Check sheet for the modelled part. Datum: model origin and axes. Units: mm. A direction names the side the tool comes from. Give positions to 0.01 mm unless a question says otherwise; leave off trailing zeros. Write each loop counter-clockwise with the first axis right and the second up, starting at its lowest first coordinate (ties: lowest second). Pieces come first, ordered by that corner, then holes. Notation, with made-up numbers: M -18.75,-3.75 L 19.25,-3.75 A15 ccw 19.25,16.25 Z; hole C 65.25,34 d3. An arc over 180 degrees is marked long. Use CSV: the item, a comma, the result in double quotes. Start each with the question number.
1. Cross-section at A-A, the plane x = 5. Enter the section's corners in (y, z).
2. Access from +Z, -Z, +X, -X, +Y, -Y to the whole of each face (thin tool, end or side, straight path). Record for faces 1 (the face through (-151.18, 125.16, 2.81)), 2 (the face through (102.025, -153, 5)), 3 (the face through (-92.04, 60.52, 4.93)).
3. Scan lines: line 1 (X direction, y = -133.5, z = 7) (3 decimals); line 2 (X direction, y = -141, z = 7.25) (3 decimals); line 3 (X direction, y = 192, z = 1) (3 decimals). Record each from-to range of solid material in increasing order.
4. Depth check by flat-ended pin: P1, Ø2, axis at x = -58.5, z = 9, coming from the +Y side; P2, Ø3.5, axis at x = -117.025, z = 5, coming from the -Y side; P3, Ø8.5, axis at x = 148.52, y = -141, coming from the -Z side. Enter the tip coordinate at first touch or a pass-through.
from build123d import *

# Parameters (mm, degrees)
SALIENTE_EXTRUIR1_DEPTH                              = 10
PERFORADOR_PARA_ROSCAR_PARA_MACHO_DE_2_COUNT         = 2
PERFORADOR_PARA_ROSCAR_PARA_MACHO_DE_2_PITCH         = 50
PERFORADOR_PARA_ROSCAR_PARA_MACHO_DE_3_COUNT         = 2
PERFORADOR_PARA_ROSCAR_PARA_MACHO_DE_3_PITCH         = 114.274917137
PERFORADOR_PARA_ROSCAR_PARA_MACHO_DE_4_COUNT         = 2
PERFORADOR_PARA_ROSCAR_PARA_MACHO_DE_4_PITCH         = 25
PERFORADOR_PARA_ROSCAR_PARA_MACHO_DE_5_A_COUNT       = 2
PERFORADOR_PARA_ROSCAR_PARA_MACHO_DE_5_A_PITCH       = 50
PERFORADOR_PARA_ROSCAR_PARA_MACHO_DE_6_COUNT         = 2
PERFORADOR_PARA_ROSCAR_PARA_MACHO_DE_6_PITCH         = 24.875395913
REFRENTADO_PARA_TORNILLO_TAP_N_CON_CABEZ_D           = 5.3
REFRENTADO_PARA_TORNILLO_TAP_N_CON_CABEZ_CSINK_D     = 11.2
REFRENTADO_PARA_TORNILLO_TAP_N_CON_CABEZ_CSINK_ANGLE = 90
SIMETR_A3_COPY_1_D                                   = 5.3
SIMETR_A3_COPY_1_CSINK_D                             = 11.2
SIMETR_A3_COPY_1_CSINK_ANGLE                         = 90
CORTAR_EXTRUIR1_DEPTH                                = 286.71506895
CORTAR_EXTRUIR1_DEPTH_BACK                           = 286.71506895
CROQUIS8_R                                           = 4


with BuildPart() as part:
    # Croquis1 → Saliente-Extruir1 (new body)
    with BuildSketch(Plane.XY):
        with BuildLine():
            Line((-67.025, 50), (67.025, 50))
            ThreePointArc((67.025, 50), (91.773737342, 60.251262658), (102.025, 85))
            Line((102.025, 85), (102.025, 220))
            Line((102.025, 220), (182.025, 220))
            Line((182.025, 220), (182.025, 60))
            Line((182.025, 60), (182.025, -60))
            Line((182.025, -60), (182.025, -220))
            Line((182.025, -220), (102.025, -220))
            Line((102.025, -220), (102.025, -85))
            ThreePointArc((102.025, -85), (91.773737342, -60.251262658), (67.025, -50))
            Line((67.025, -50), (-67.025, -50))
            ThreePointArc((-67.025, -50), (-91.773737342, -60.251262658), (-102.025, -85))
            Line((-102.025, -85), (-102.025, -220))
            Line((-102.025, -220), (-182.025, -220))
            Line((-182.025, -220), (-182.025, -60))
            Line((-182.025, -60), (-182.025, 60))
            Line((-182.025, 60), (-182.025, 220))
            Line((-182.025, 220), (-102.025, 220))
            Line((-102.025, 220), (-102.025, 85))
            ThreePointArc((-102.025, 85), (-91.773737342, 60.251262658), (-67.025, 50))
        make_face()
    extrude(amount=SALIENTE_EXTRUIR1_DEPTH)

    # Croquis3 → Perforador para roscar para macho de ros (revolve, cut)
    with BuildSketch(Plane(origin=(-167.025, 220, 5), x_dir=(0, 0, 1), z_dir=(1, 0, 0))):
        Polygon((0, 0), (0, 76.2618073), (2.1, 75), (2.1, 0), align=None)
    perforador_para_roscar_para_macho_de_ros = revolve(axis=Axis((-167.025, 226.35, 5), (0, -1, 0)), mode=Mode.SUBTRACT)

    # Perforador para roscar para macho de 2: Perforador para roscar para macho de ros ×2
    with Locations(*[(i * PERFORADOR_PARA_ROSCAR_PARA_MACHO_DE_2_PITCH, 0, 0) for i in range(1, PERFORADOR_PARA_ROSCAR_PARA_MACHO_DE_2_COUNT)]):
        add(perforador_para_roscar_para_macho_de_ros, mode=Mode.SUBTRACT)

    # Perforador para roscar para macho de 3: Perforador para roscar para macho de ros ×2
    with Locations(*[Vector(-0.9105437359751597, 0, -0.4134127536450694) * (i * PERFORADOR_PARA_ROSCAR_PARA_MACHO_DE_3_PITCH) for i in range(1, PERFORADOR_PARA_ROSCAR_PARA_MACHO_DE_3_COUNT)]):
        add(perforador_para_roscar_para_macho_de_ros, mode=Mode.SUBTRACT)

    # Perforador para roscar para macho de 4: Perforador para roscar para macho de ros ×2
    with Locations(*[(i * PERFORADOR_PARA_ROSCAR_PARA_MACHO_DE_4_PITCH, 0, 0) for i in range(1, PERFORADOR_PARA_ROSCAR_PARA_MACHO_DE_4_COUNT)]):
        add(perforador_para_roscar_para_macho_de_ros, mode=Mode.SUBTRACT)

    # Croquis5 → Perforador para roscar para macho de 5 (revolve, cut)
    with BuildSketch(Plane(origin=(117.025, 220, 5), x_dir=(0, 0, 1), z_dir=(1, 0, 0))):
        Polygon((0, 0), (0, 76.2618073), (2.1, 75), (2.1, 0), align=None)
    perforador_para_roscar_para_macho_de_5 = revolve(axis=Axis((117.025, 226.35, 5), (0, -1, 0)), mode=Mode.SUBTRACT)

    # Perforador para roscar para macho de 5 a: Perforador para roscar para macho de 5 ×2
    with Locations(*[(i * PERFORADOR_PARA_ROSCAR_PARA_MACHO_DE_5_A_PITCH, 0, 0) for i in range(1, PERFORADOR_PARA_ROSCAR_PARA_MACHO_DE_5_A_COUNT)]):
        add(perforador_para_roscar_para_macho_de_5, mode=Mode.SUBTRACT)

    # Perforador para roscar para macho de 6: Perforador para roscar para macho de 5 ×2
    with Locations(*[Vector(0.9999846303252095, 0, 0.005544286550521713) * (i * PERFORADOR_PARA_ROSCAR_PARA_MACHO_DE_6_PITCH) for i in range(1, PERFORADOR_PARA_ROSCAR_PARA_MACHO_DE_6_COUNT)]):
        add(perforador_para_roscar_para_macho_de_5, mode=Mode.SUBTRACT)

    # Simetría1: Perforador para roscar para macho de ros, Perforador para roscar para macho de 5 across plane
    add(perforador_para_roscar_para_macho_de_ros.mirror(Plane.ZX), mode=Mode.SUBTRACT)
    add(perforador_para_roscar_para_macho_de_5.mirror(Plane.ZX), mode=Mode.SUBTRACT)

    # Simetría1 copy 1 sketch → Simetría1 copy 1 (revolve, cut)
    with BuildSketch(Plane(origin=(-117.025, -220, 5), x_dir=(0, 0, 1), z_dir=(1, 0, 0))):
        Polygon((0, 0), (0, -76.2618073), (2.1, -75), (2.1, 0), align=None)
    revolve(axis=Axis((-117.025, -226.35, 5), (0, -1, 0)), mode=Mode.SUBTRACT)

    # Simetría1 copy 2 sketch → Simetría1 copy 2 (revolve, cut)
    with BuildSketch(Plane(origin=(-271.077309978, -220, -42.242708166), x_dir=(0, 0, 1), z_dir=(1, 0, 0))):
        Polygon((0, 0), (0, -76.2618073), (2.1, -75), (2.1, 0), align=None)
    revolve(axis=Axis((-271.077309978, -226.35, -42.242708166), (0, -1, 0)), mode=Mode.SUBTRACT)

    # Simetría1 copy 3 sketch → Simetría1 copy 3 (revolve, cut)
    with BuildSketch(Plane(origin=(-142.025, -220, 5), x_dir=(0, 0, 1), z_dir=(1, 0, 0))):
        Polygon((0, 0), (0, -76.2618073), (2.1, -75), (2.1, 0), align=None)
    revolve(axis=Axis((-142.025, -226.35, 5), (0, -1, 0)), mode=Mode.SUBTRACT)

    # Simetría1 copy 4 sketch → Simetría1 copy 4 (revolve, cut)
    with BuildSketch(Plane(origin=(167.025, -220, 5), x_dir=(0, 0, 1), z_dir=(1, 0, 0))):
        Polygon((0, 0), (0, -76.2618073), (2.1, -75), (2.1, 0), align=None)
    revolve(axis=Axis((167.025, -226.35, 5), (0, -1, 0)), mode=Mode.SUBTRACT)

    # Simetría1 copy 5 sketch → Simetría1 copy 5 (revolve, cut)
    with BuildSketch(Plane(origin=(141.900013587, -220, 5.137916323), x_dir=(0, 0, 1), z_dir=(1, 0, 0))):
        Polygon((0, 0), (0, -76.2618073), (2.1, -75), (2.1, 0), align=None)
    revolve(axis=Axis((141.900013587, -226.35, 5.137916323), (0, -1, 0)), mode=Mode.SUBTRACT)

    # Refrentado para tornillo tapón con cabeza plana de clavija de M51 (through all)
    with Locations(Plane(origin=(148.520190528, -141, 0), x_dir=(-1, 0, 0), z_dir=(0, 0, -1))):
        with Locations((0, 0), (12.990381056, 7.5), (12.990381056, -7.5), (0, 15)):
            refrentado_para_tornillo_tap_n_con_cabez = CounterSinkHole(REFRENTADO_PARA_TORNILLO_TAP_N_CON_CABEZ_D / 2, REFRENTADO_PARA_TORNILLO_TAP_N_CON_CABEZ_CSINK_D / 2, counter_sink_angle=REFRENTADO_PARA_TORNILLO_TAP_N_CON_CABEZ_CSINK_ANGLE)

    # Simetría2: Refrentado para tornillo tapón con cabeza plana de clavija de M51 across plane
    add(refrentado_para_tornillo_tap_n_con_cabez.mirror(Plane.ZX), mode=Mode.SUBTRACT)

    # Simetría3: Refrentado para tornillo tapón con cabeza plana de clavija de M51 across plane
    add(refrentado_para_tornillo_tap_n_con_cabez.mirror(Plane(origin=(0, 0, 0), x_dir=(0, 0, 1), z_dir=(1, 0, 0))), mode=Mode.SUBTRACT)

    # Simetría3 copy 1 (through all)
    with Locations(Plane(origin=(-148.520190528, 141, 0), x_dir=(1, 0, 0), z_dir=(0, 0, -1))):
        with Locations((0, 0), (12.990381056, 7.5), (12.990381056, -7.5), (0, 15)):
            CounterSinkHole(SIMETR_A3_COPY_1_D / 2, SIMETR_A3_COPY_1_CSINK_D / 2, counter_sink_angle=SIMETR_A3_COPY_1_CSINK_ANGLE)

    # Croquis8 → Cortar-Extruir1 (cut, two sides: drawn at the far end of the back side and taken through both)
    with BuildSketch(Plane.XY.offset(10).offset(-CORTAR_EXTRUIR1_DEPTH_BACK)):
        with Locations((167.025, 0)):
            Circle(CROQUIS8_R)
        with Locations((-159.025, 0)):
            Circle(CROQUIS8_R)
    extrude(amount=CORTAR_EXTRUIR1_DEPTH + CORTAR_EXTRUIR1_DEPTH_BACK, mode=Mode.SUBTRACT)


solid = part.part
Worked answers:
1,outline,"M -50,0 L 50,0 L 50,10 L -50,10 Z"
2,face 1,"-Z"
2,face 2,"+Z, -Z, -Y"
2,face 3,"+Z, -Z, +Y"
3,line 1,"x = -182.025 to -138.18, -132.88 to -102.025, 102.025 to 132.88, 138.18 to 182.025"
3,line 2,"x = -182.025 to -151.17, -145.87 to -102.025, 102.025 to 145.87, 151.17 to 182.025"
3,line 3,"x = -182.025 to -102.025, 102.025 to 182.025"
4,P1,"stops at y = 50"
4,P2,"stops at y = -144.79"
4,P3,"stops at z = 1.35"
